CAD build for the part. Positions are in the model's coordinates, mm. A direction names the side the tool comes from. Coordinates: 2 decimals unless noted, no trailing zeros. Loops run counter-clockwise (first coordinate to the right, second up) from the corner with the lowest first, then second, coordinate; pieces in that order, holes last. Notation, with made-up numbers: (-23, 89.5) -> (31, 89.5) arc R23 cw to (31, 116.5) -> close; hole circle Ø1 at (26.5, 9.25). An arc over 180 degrees is marked (long way). Write each question's results on one line, items separated by ' | '.
```python
from build123d import *

# Parameters (mm, degrees)
SALIENTE_EXTRUIR1_DEPTH = 3
REDONDEO1_R             = 10
CROQUIS2_R              = 1.5
CROQUIS2_R_2            = 1.55
CORTAR_EXTRUIR1_DEPTH   = 135.610141171
CROQUIS4_W              = 110
CROQUIS4_H              = 50
CORTAR_EXTRUIR2_DEPTH   = 135.610141171
REDONDEO2_R             = 5
CROQUIS5_W              = 4
CROQUIS5_H              = 14.636342218
CORTAR_EXTRUIR3_DEPTH   = 135.610141171
CROQUIS6_W              = 14.636342218
CROQUIS6_H              = 3
SALIENTE_EXTRUIR2_DEPTH = 2
CROQUIS8_W              = 14.636342218
CROQUIS8_H              = 3
SALIENTE_EXTRUIR3_DEPTH = 2
CROQUIS9_W              = 196.2
CROQUIS9_H              = 31.087527503
CORTAR_EXTRUIR4_DEPTH   = 133.713564137
CROQUIS10_R             = 2
CORTAR_EXTRUIR5_DEPTH   = 133.713564137
REDONDEO6_R             = 15
CROQUIS11_R             = 2
CORTAR_EXTRUIR6_DEPTH   = 10


with BuildPart() as part:
    # Croquis1 → Saliente-Extruir1 (new body)
    with BuildSketch(Plane(origin=(0, 0, 0), x_dir=(1, 0, 0), z_dir=(0, 1, 0))):
        Polygon((-88.1, 42.318171109), (88.1, 42.318171109), (108.1, 22.318171109), (127.75, 22.318171109), (127.75, 7.681828891), (105.75, 7.681828891), (77.75, -42.318171109), (-77.75, -42.318171109), (-105.75, 7.681828891), (-127.75, 7.681828891), (-127.75, 22.318171109), (-108.1, 22.318171109), align=None)
    extrude(amount=SALIENTE_EXTRUIR1_DEPTH)

    # Redondeo1
    redondeo1_edges = [part.edges().sort_by_distance(p)[0] for p in [
        (-88.1, 1.5, -42.318171109),
        (88.1, 1.5, -42.318171109),
        (108.1, 1.5, -22.318171109),
        (105.75, 1.5, -7.681828891),
        (77.75, 1.5, 42.318171109),
        (-77.75, 1.5, 42.318171109),
        (-105.75, 1.5, -7.681828891),
        (-108.1, 1.5, -22.318171109),
    ]]
    fillet(redondeo1_edges, radius=REDONDEO1_R)

    # Croquis2 → Cortar-Extruir1 (cut, through all)
    with BuildSketch(Plane(origin=(0, 3, 0), x_dir=(1, 0, 0), z_dir=(0, 1, 0))):
        with Locations(Location((70, -27.318171109, 0), (0, 0, 270))):
            Circle(CROQUIS2_R)
        with Locations(Location((-70, -27.318171109, 0), (0, 0, 270))):
            Circle(CROQUIS2_R)
        with Locations(Location((-119.996067812, 15, 0), (0, 0, 270))):
            Circle(CROQUIS2_R_2)
        with Locations(Location((119.996067812, 15, 0), (0, 0, 270))):
            Circle(CROQUIS2_R_2)
        with Locations(Location((-17.5, -17.318171109, 0), (0, 0, 270))):
            Circle(CROQUIS2_R)
        with Locations(Location((17.5, -17.318171109, 0), (0, 0, 270))):
            Circle(CROQUIS2_R)
        with Locations(Location((-17.5, -37.318171109, 0), (0, 0, 270))):
            Circle(CROQUIS2_R)
        with Locations(Location((17.5, -37.318171109, 0), (0, 0, 270))):
            Circle(CROQUIS2_R)
    extrude(amount=-CORTAR_EXTRUIR1_DEPTH, mode=Mode.SUBTRACT)

    # Croquis4 → Cortar-Extruir2 (cut, through all)
    with BuildSketch(Plane(origin=(0, 3, 0), x_dir=(1, 0, 0), z_dir=(0, 1, 0))):
        with Locations((0, -17.318171109)):
            Rectangle(CROQUIS4_W, CROQUIS4_H)
    extrude(amount=-CORTAR_EXTRUIR2_DEPTH, mode=Mode.SUBTRACT)

    # Redondeo2
    redondeo2_edges = [part.edges().sort_by_distance(p)[0] for p in [
        (55, 1.5, 42.318171109),
        (-55, 1.5, 42.318171109),
        (-55, 1.5, -7.681828891),
        (55, 1.5, -7.681828891),
    ]]
    fillet(redondeo2_edges, radius=REDONDEO2_R)

    # Croquis5 → Cortar-Extruir3 (cut, through all)
    with BuildSketch(Plane(origin=(0, 3, 0), x_dir=(1, 0, 0), z_dir=(0, 1, 0))):
        with Locations((-125.75, 15)):
            Rectangle(CROQUIS5_W, CROQUIS5_H)
        with Locations((125.75, 15)):
            Rectangle(CROQUIS5_W, CROQUIS5_H)
    extrude(amount=-CORTAR_EXTRUIR3_DEPTH, mode=Mode.SUBTRACT)

    # Croquis6 → Saliente-Extruir2 (add)
    with BuildSketch(Plane(origin=(123.75, 0, 0), x_dir=(0, 0, -1), z_dir=(1, 0, 0))):
        with Locations((15, 1.5)):
            Rectangle(CROQUIS6_W, CROQUIS6_H)
    extrude(amount=SALIENTE_EXTRUIR2_DEPTH)

    # Croquis8 → Saliente-Extruir3 (add)
    with BuildSketch(Plane.ZY.offset(123.75)):
        with Locations((-15, 1.5)):
            Rectangle(CROQUIS8_W, CROQUIS8_H)
    extrude(amount=SALIENTE_EXTRUIR3_DEPTH)

    # Croquis9 → Cortar-Extruir4 (cut, through all)
    with BuildSketch(Plane(origin=(0, 3, 0), x_dir=(1, 0, 0), z_dir=(0, 1, 0))):
        with Locations((0, 50.861934861)):
            Rectangle(CROQUIS9_W, CROQUIS9_H)
    extrude(amount=-CORTAR_EXTRUIR4_DEPTH, mode=Mode.SUBTRACT)

    # Croquis10 → Cortar-Extruir5 (cut, through all)
    with BuildSketch(Plane(origin=(0, 3, 0), x_dir=(1, 0, 0), z_dir=(0, 1, 0))):
        with Locations(Location((-52.5, 27.318171109, 0), (0, 0, 270))):
            Circle(CROQUIS10_R)
        with Locations(Location((52.5, 27.318171109, 0), (0, 0, 270))):
            Circle(CROQUIS10_R)
    extrude(amount=-CORTAR_EXTRUIR5_DEPTH, mode=Mode.SUBTRACT)

    # Redondeo6
    redondeo6_edges = [part.edges().sort_by_distance(p)[0] for p in [
        (-95.1, 1.5, -35.318171109),
        (95.1, 1.5, -35.318171109),
    ]]
    fillet(redondeo6_edges, radius=REDONDEO6_R)

    # Croquis11 → Cortar-Extruir6 (cut)
    with BuildSketch(Plane(origin=(0, 3, 0), x_dir=(1, 0, 0), z_dir=(0, 1, 0))):
        with Locations(Location((-62.1, -35.218171109, 0), (0, 0, 270))):
            Circle(CROQUIS11_R)
        with Locations(Location((62.1, -35.218171109, 0), (0, 0, 270))):
            Circle(CROQUIS11_R)
    extrude(amount=-CORTAR_EXTRUIR6_DEPTH, mode=Mode.SUBTRACT)


solid = part.part
```
Q1. Pull direction X, two halves, no side cores. Call faces 1 (the flat face through (2, 0, -14)), 2 (the flat face through (91.906, 1.479, 17.04)), 3 (the flat face through (-91.59, 1.48, 17.6)), 4 (the cylindrical face through (-53.57, 1.48, -6.18)): +X half, -X half, draft (parallel to the pull), parting line (faces both ways), or undercut.
Results are:
face 1: draft | face 2: +X half | face 3: -X half | face 4: undercut
Q2. Cut at B-B on x = -23. Write the cut outline in (y, z), and give its area (3 significant figures).
Results are:
outline: (0, -35.32) -> (3, -35.32) -> (3, -7.68) -> (0, -7.68) -> close | area: 82.9 mm^2
Q3. Cut at D-D on x = 77. Write the cut outline in (y, z), and give its area (3 significant figures).
Results are:
outline: (0, -35.32) -> (3, -35.32) -> (3, 40.91) -> (0, 40.91) -> close | area: 229 mm^2
Q4. Which spindle directions (+Z, -Z, +X, -X, +Y, -Y) get a long thin tool onto all of the face, cutting with end or side? Do faces 5 (the cylindrical face through (56.426, 1.479, 40.815)), 6 (the flat face through (2, 3, -14)). Say none if no direction does.
Results are:
face 5: +Z, +Y, -Y | face 6: +Z, -Z, +X, -X, +Y
Q5. Wall check: L1, parallel to X at y = 1.95, z = -15; L2, parallel to Z at x = -70, y = 1.15; L3, parallel to X at y = 2.15, z = 34. Give the ranges that are in metal, low to high. Write a range as from..to.
Results are:
L1: -125.75..-121.55, -118.45..118.45, 121.55..125.75 | L2: -35.32..25.82, 28.82..42.32 | L3: -82.41..-63.69, -60.51..-55, 55..60.51, 63.69..82.41
Q6. Cut at C-C on y = 1.45. Give the number of separate pieces and of enclosed holes in the cut face, and give its area (3 significant figures).
Results are:
separate pieces: 1 | enclosed holes: 8 | area: 9,910 mm^2
Q7. Drop flat-ended pins along their axis: pin 1 (0.9 mm diameter, centred on x = 121, y = 1, fed in from -Z); pin 2 (3.5 mm diameter, centred on x = 62.1, z = 35.22, fed in from -Y); pin 3 (0.9 mm diameter, centred on y = 2, z = 19.5, fed in from -X); pin 4 (0.9 mm diameter, centred on y = 1, z = 11, fed in from +X). Give the stop position or say it passes through.
Results are:
pin 1: z = -22.32 | pin 2: through | pin 3: x = -90.78 | pin 4: x = 95.54
Q8. Cut at A-A on z = -5. Write the cut outline in (x, y).
Results are:
outline: (-104.8, 0) -> (-54.43, 0) -> (-54.43, 3) -> (-104.8, 3) -> close; (54.43, 0) -> (104.8, 0) -> (104.8, 3) -> (54.43, 3) -> close
